Design review of the part shown in the three views and the two pictorial views. Dimensions are in mm from the part's minimum x, y and z. A direction names the side the tool comes from. Coordinates: 2 decimals unless noted, no trailing zeros. Loops run counter-clockwise (first coordinate to the right, second up) from the corner with the lowest first, then second, coordinate; pieces in that order, holes last. Notation, with made-up numbers: M 12,21 L 31,21 A12 cw 31,30 Z; hole C 73,60.5 d11. An arc over 180 degrees is marked long. Use one line per item in the form item = value.
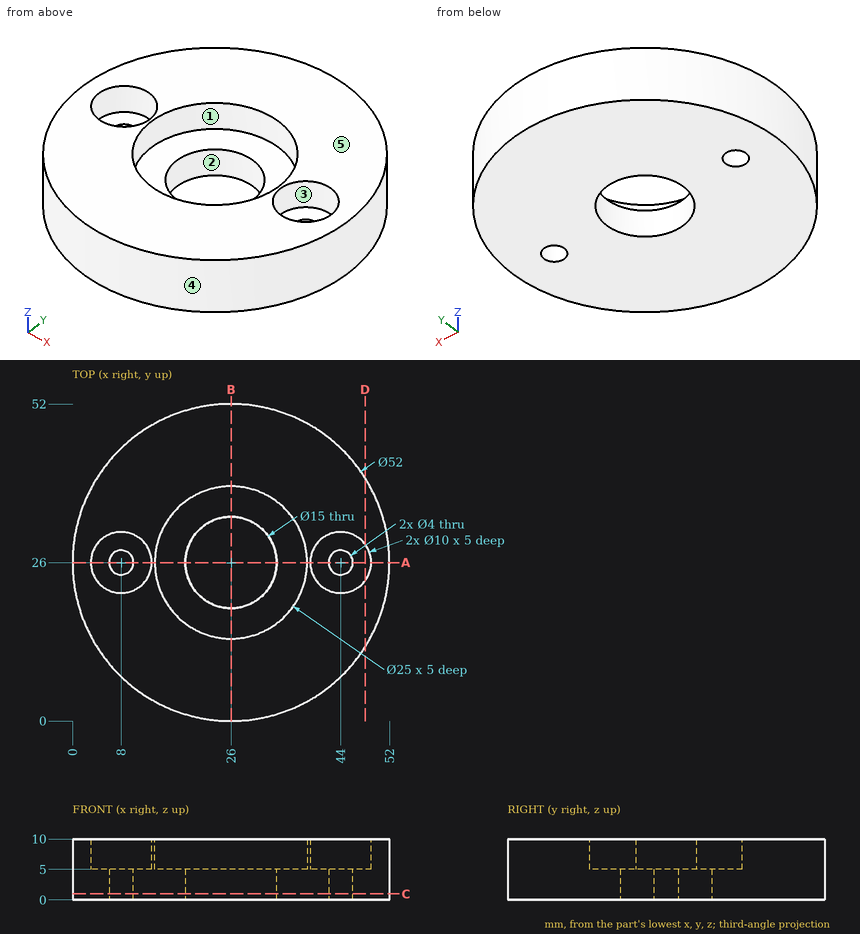
1. The part is to be moulded in two halves that separate along Y. For the marked faces 3, 4 and 5, say which applies: pulls with the +Y half, pulls with the -Y half, needs draft (parallel to the pull), parting line crosses it, or undercut.
Response values:
face_3 = undercut
face_4 = parting line crosses it
face_5 = needs draft
2. Wall thickness on line 1 along X through (y, z) = (25, 7.25); line 2 along Z through (x, y) = (43, 29); line 3 along X through (y, z) = (22, 7): over which ranges is each line inside the solid? List them lowest first. Write a range as from..to.
Response values:
line_1 = 0.02..3.1, 12.9..13.54, 38.46..39.1, 48.9..51.98
line_2 = 0..5
line_3 = 0.31..5, 11..14.16, 37.84..41, 47..51.69
3. Machinability: for the marked faces 1 and 2, which of the approach directions +Z, -Z, +X, -X, +Y, -Y give a long, thin tool a straight path to every point of the face, cutting with its end or side? Answer none if there is none.
Response values:
face_1 = +Z
face_2 = +Z, -Z
4. Add section B-B (x = 26). State the section outline as (y, z) points.
Response values:
outline = M 0,0 L 18.5,0 L 18.5,5 L 13.5,5 L 13.5,10 L 0,10 Z; M 33.5,0 L 52,0 L 52,10 L 38.5,10 L 38.5,5 L 33.5,5 Z
5. Insertion check: P1, Ø2.5, axis at x = 44, y = 26, coming from the +Z side; P2, Ø24, axis at x = 26, y = 26, coming from the -Z side; P3, Ø5, axis at y = 47, z = 8, coming from the +X side; P4, Ø1, axis at x = 11, z = 6.5, coming from the +Y side. Each pin has a flat end and moves straight along its axis. Give the tip position at first contact, or say it passes through.
Response values:
P1 = through
P2 = 0
P3 = 44.27
P4 = 47.58
6. Add section C-C (z = 1). State the section outline as (x, y) points, then the cut area to 3 significant figures.
Response values:
outline = C 26,26 d52; hole C 8,26 d4; hole C 26,26 d15; hole C 44,26 d4
area = 1,920 mm^2
7. Add section A-A (y = 26). State the section outline as (x, z) points.
Response values:
outline = M 0,0 L 6,0 L 6,5 L 3,5 L 3,10 L 0,10 Z; M 10,0 L 18.5,0 L 18.5,5 L 13.5,5 L 13.5,10 L 13,10 L 13,5 L 10,5 Z; M 33.5,0 L 42,0 L 42,5 L 39,5 L 39,10 L 38.5,10 L 38.5,5 L 33.5,5 Z; M 46,0 L 52,0 L 52,10 L 49,10 L 49,5 L 46,5 Z
8. Add section D-D (x = 48). State the section outline as (y, z) points, then the cut area to 3 significant figures.
Response values:
outline = M 12.14,0 L 39.86,0 L 39.86,10 L 29,10 L 29,5 L 23,5 L 23,10 L 12.14,10 Z
area = 247 mm^2
